Verification items for this drawing (mm, ordinates from the low corner). Round coordinates to 2 decimals unless told otherwise and drop trailing zeros. Loops run counter-clockwise (first coordinate to the right, second up) from the corner with the lowest first, then second, coordinate; pieces in that order, holes last. Notation, with made-up numbers: M -24,82.5 L -9,82.5 A14 ccw -9,90.5 Z; hole C -39.75,16 d10. An arc over 180 degrees is marked long. Write item = value, one per line. Start each with the question number.
(1) Mould release check, pull along X, two halves, no side actions. Record for the marked faces 1, 2 and 3: pulls with the +X half, pulls with the -X half, needs draft (parallel to the pull), parting line crosses it, or undercut.
(2) Cross-section at C-C on x = 220. Record the boundary of the cut face in (y, z), plus the area to 3 significant figures.
(3) Cross-section at A-A on y = 19.05. Record the boundary of the cut face in (x, z), plus the area to 3 significant figures.
(4) Scan lines: L1, parallel to Z at x = 259, y = 19; L2, parallel to Z at x = 20.5, y = 19.5; L3, parallel to Y at x = 311.5, z = 31. Record each from-to range of solid material in increasing order. Write a range as from..to.
(5) Go/stop test with flat-tipped pins: P1, Ø1.5, axis at x = 232.5, y = 24.5, coming from the +Z side; P2, Ø6.5, axis at x = 349.5, z = 25, coming from the -Y side; P3, Ø5, axis at x = 209.5, y = 28.5, coming from the -Z side. Record where each tip stops, or that it passes through.
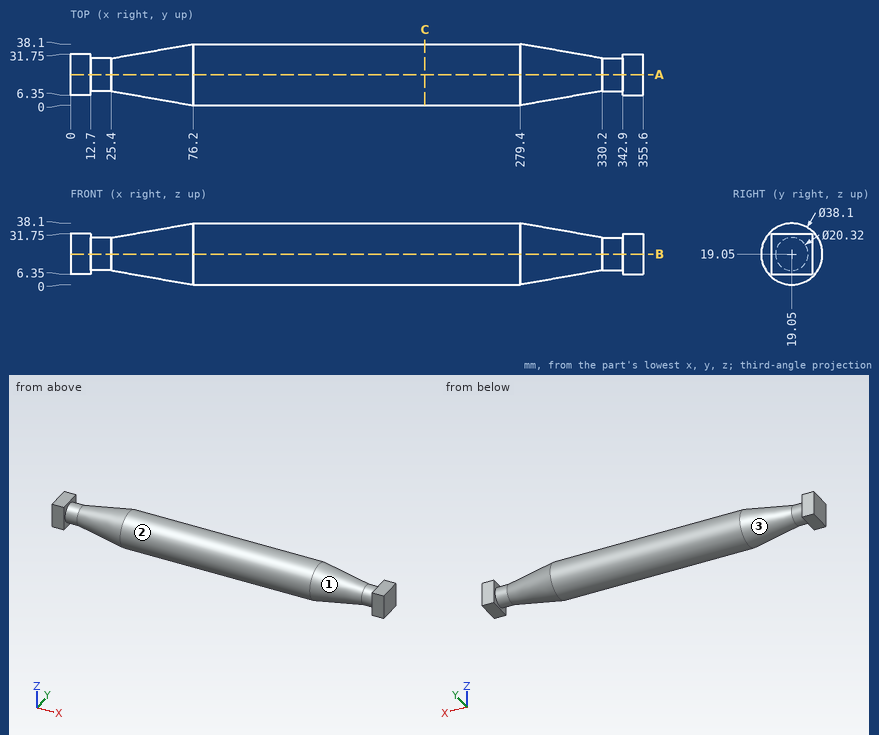
Result:
q1.face_1 = undercut
q1.face_2 = needs draft
q1.face_3 = undercut
q2.outline = C 19.05,19.05 d38.1
q2.area = 1,140 mm^2
q3.outline = M 0,6.35 L 12.7,6.35 L 12.7,8.89 L 25.4,8.89 L 76.2,0 L 279.4,0 L 330.2,8.89 L 342.9,8.89 L 342.9,6.35 L 355.6,6.35 L 355.6,31.75 L 342.9,31.75 L 342.9,29.21 L 330.2,29.21 L 279.4,38.1 L 76.2,38.1 L 25.4,29.21 L 12.7,29.21 L 12.7,31.75 L 0,31.75 Z
q3.area = 11,900 mm^2
q4.L1 = 0..38.1
q4.L2 = 8.9..29.2
q4.L3 = 12.92..25.18
q5.P1 = 37.51
q5.P2 = 6.35
q5.P3 = 1.31
